Geometry check sheet. Reference: the model listing, model coordinates, mm. Face numbers are marked on the shaded views. A direction names the side the tool comes from. Give positions to 0.01 mm unless a question says otherwise; leave off trailing zeros. Order: outer loops, then holes, each group sorted by start corner. A loop starts at its lowest first (then second) coordinate and runs counter-clockwise, first axis right, second up. Notation, with made-up numbers: M 10,8 L 27,8 A24 cw 27,32 Z; hole C -18,37.25 d7. An arc over 180 degrees is marked long. One line per question, with ' | ' between items. Start each with the question number.
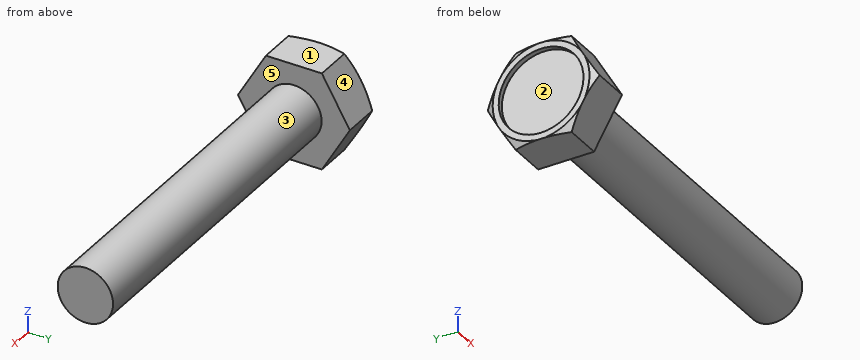
from build123d import *

# Parameters (mm, degrees)
SKETCH2_R     = 4.081986143
HEX_DIE_DEPTH = 3
SKETCH4_R     = 3.0625
INDENT_DEPTH  = 0.375


with BuildPart() as part:
    # BodySke → Base-Revolve (revolve)
    with BuildSketch(Plane.XY):
        Polygon((3, 2), (3, 4.041570439), (0.312675839, 4.041570439), (0, 3.5), (0, 0), (28, 0), (28, 2), align=None)
    revolve(axis=Axis((-25.4, 0, 0), (1, 0, 0)))

    # Sketch2 → Hex-Die (cut)
    with BuildSketch(Plane(origin=(0, 0, 0), x_dir=(0, 0, -1), z_dir=(1, 0, 0))):
        Circle(SKETCH2_R)
        Polygon((-3.5, 2.020725951), (0, 4.041451902), (3.5, 2.020725951), (3.5, -2.020725951), (0, -4.041451902), (-3.5, -2.020725951), align=None, mode=Mode.SUBTRACT)
    extrude(amount=HEX_DIE_DEPTH, mode=Mode.SUBTRACT)

    # Sketch4 → Indent (cut)
    with BuildSketch(Plane(origin=(0, 0, 0), x_dir=(0, 0, -1), z_dir=(1, 0, 0))):
        Circle(SKETCH4_R)
    extrude(amount=INDENT_DEPTH, mode=Mode.SUBTRACT)


solid = part.part
Item 1: Depth check by flat-ended pin: pin 1 (1 mm diameter, centred on y = -1, z = -2, fed in from -X) (3 decimals); pin 2 (3 mm diameter, centred on y = 2.5, z = 1.5, fed in from +X); pin 3 (3 mm diameter, centred on x = 21.5, y = 1, fed in from +Z). Enter the tip coordinate at first touch or a pass-through.
Item 2: Material ranges on line 1 along X through (y, z) = (-0.25, 3) (3 decimals); line 2 along Y through (x, z) = (0.15, 0); line 3 along X through (y, z) = (-1.25, -3), recorded low to high.
Item 3: Cross-section at A-A, the plane x = 9.25. Record the cut outline in (y, z), plus the area to 3 significant figures.
Item 4: Set-up check for the marked faces 4 and 5: record each of +Z, -Z, +X, -X, +Y, -Y from which the full face is reachable in a straight line by a thin tool's end or side.
Item 5: Mould release check, pull along Z, two halves, no side actions. Record for the marked faces 1, 2 and 3: released by +Z, released by -Z, zero draft, split by the parting line, or undercut.
Outcome:
1) pin 1: stops at x = 0.375 | pin 2: stops at x = 28 | pin 3: stops at z = 2
2) line 1: x = 0.375 to 3 | line 2: y = -3.76 to -3.06, 3.06 to 3.76 | line 3: x = 0 to 3
3) outline: C 0,0 d4 | area: 12.6 mm²
4) face 4: +Z, +X, -X, +Y | face 5: +X
5) face 1: released by +Z | face 2: undercut | face 3: split by the parting line
